Check sheet for the drawn part. Datum: minimum x, y, z corner. Units: mm. Coordinates: 2 decimals unless noted, no trailing zeros. Loops run counter-clockwise (first coordinate to the right, second up) from the corner with the lowest first, then second, coordinate; pieces in that order, holes last. Notation, with made-up numbers: (25.25, -26.5) - (39.25, -26.5) arc R32 ccw to (39.25, 6.5) - close; hole circle Ø5 at (-14, -2.5). An arc over 180 degrees is marked (long way). Answer as a JSON object with one key per item and string values. Group by question number.
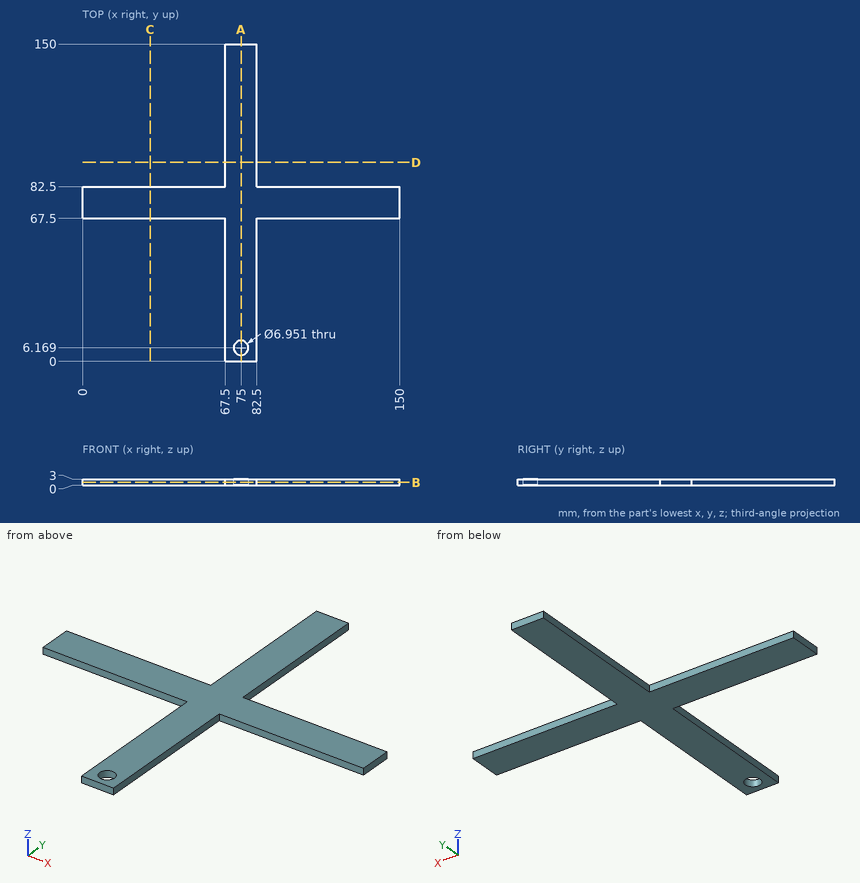
1. Sectioned sample at C-C on x = 32. Record the cut outline in (y, z), plus the area to 3 significant figures.
2. Material ranges on line 1 (Y direction, x = 75, z = 1.7) (1 decimal); line 2 (Y direction, x = 88, z = 1.7), recorded low to high.
3. Sectioned sample at A-A on x = 75. Record the cut outline in (y, z) (1 decimal), plus the area to 3 significant figures.
4. Gauge pin test, flat ends, axial feed: pin 1 (6 mm diameter, centred on x = 73, y = 102, fed in from -Z); pin 2 (1.5 mm diameter, centred on x = 102, z = 1.5, fed in from +Y); pin 3 (4 mm diameter, centred on x = 75, y = 6.17, fed in from -Z); pin 4 (0.9 mm diameter, centred on x = 18, z = 1.5, fed in from -Y). Record the tip position at first contact, or that the pin passes through.
5. Sectioned sample at B-B on z = 1.4. Record the cut outline in (x, y).
Answers follow:
{
 "1": {"outline": "(67.5, 0) - (82.5, 0) - (82.5, 3) - (67.5, 3) - close", "area": "45.0 mm^2"},
 "2": {"line 1": "y = 0 to 2.7, 9.6 to 150", "line 2": "y = 67.5 to 82.5"},
 "3": {"outline": "(0, 0) - (2.7, 0) - (2.7, 3) - (0, 3) - close; (9.6, 0) - (150, 0) - (150, 3) - (9.6, 3) - close", "area": "429 mm^2"},
 "4": {"pin 1": "stops at z = 0", "pin 2": "stops at y = 82.5", "pin 3": "passes through", "pin 4": "stops at y = 67.5"},
 "5": {"outline": "(0, 67.5) - (67.5, 67.5) - (67.5, 0) - (82.5, 0) - (82.5, 67.5) - (150, 67.5) - (150, 82.5) - (82.5, 82.5) - (82.5, 150) - (67.5, 150) - (67.5, 82.5) - (0, 82.5) - close; hole circle Ø6.95 at (75, 6.17)"}
}
